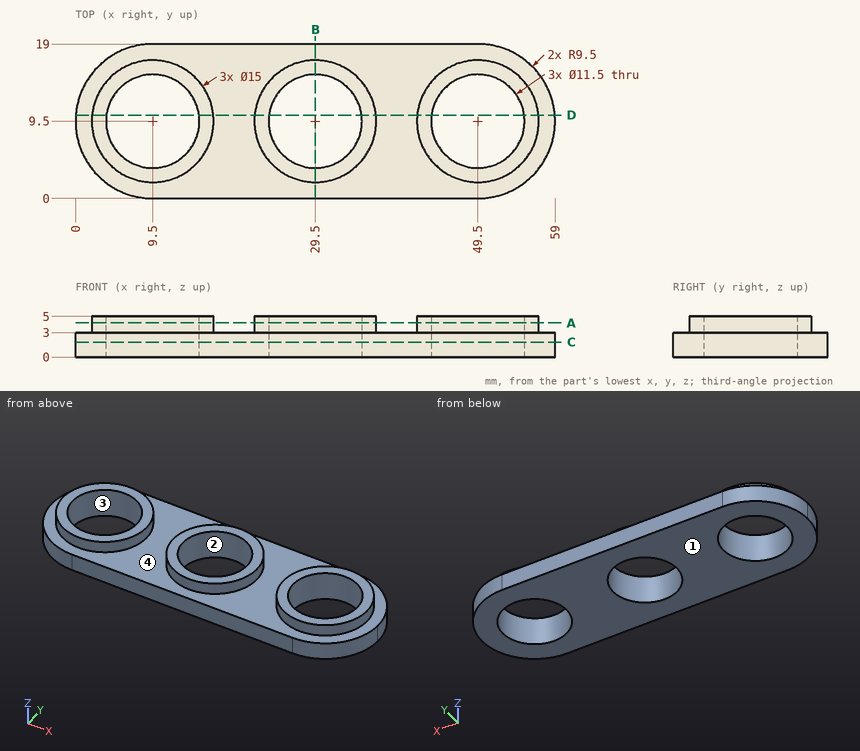
Verification items for this drawing (mm, ordinates from the low corner). A direction names the side the tool comes from. Coordinates: 2 decimals unless noted, no trailing zeros. Write each loop counter-clockwise with the first axis right and the second up, starting at its lowest first coordinate (ties: lowest second). Pieces come first, ordered by that corner, then holes. Notation, with made-up numbers: M -33.75,68.25 L 14.25,68.25 A18 ccw 14.25,78.25 Z; hole C -1,55 d11. An arc over 180 degrees is marked long. One line per item, written item: value. Start each with the question number.
(1) Depth check by flat-ended pin: pin 1 (2 mm diameter, centred on y = 9, z = 4.5, fed in from +X); pin 2 (10.5 mm diameter, centred on x = 9.5, y = 9.5, fed in from -Z); pin 3 (2 mm diameter, centred on y = 15, z = 3, fed in from -X); pin 4 (2 mm diameter, centred on y = 3, z = 3.5, fed in from +X). Enter the tip coordinate at first touch or a pass-through.
(2) Scan lines: line 1 along Y through (x, z) = (9.5, 1.6); line 2 along Y through (x, z) = (9.5, 3.3); line 3 along X through (y, z) = (8.25, 1.75). Record each from-to range of solid material in increasing order. Write a range as [from, to].
(3) Sectioned sample at B-B, the plane x = 29.5. Enter the section's corners in (y, z), and give its area (3 significant figures).
(4) Sectioned sample at A-A, the plane z = 4.2. Enter the section's corners in (x, y).
(5) Sectioned sample at D-D, the plane y = 10.25. Enter the section's corners in (x, z), and give its area (3 significant figures).
(6) Release check for a two-part mould opening along X. For the marked faces 1 and 2 record: released by +X, released by -X, zero draft, split by the parting line, or undercut.
(7) Sectioned sample at C-C, the plane z = 1.85. Enter the section's corners in (x, y), and give its area (3 significant figures).
(8) Tool access check on the marked faces 3 and 4. Record the directions out of +Z, -Z, +X, -X, +Y, -Y that give a thin tool (end or side, any length) a straight path to the whole face; none if there is none.
Filled sheet:
1. pin 1: x = 57
1. pin 2: through
1. pin 3: x = 1.13
1. pin 4: x = 57.15
2. line 1: [0, 3.75], [15.25, 19]
2. line 2: [2, 3.75], [15.25, 17]
2. line 3: [0.08, 3.89], [15.11, 23.89], [35.11, 43.89], [55.11, 58.92]
3. outline: M 0,0 L 3.75,0 L 3.75,5 L 2,5 L 2,3 L 0,3 Z; M 15.25,0 L 19,0 L 19,3 L 17,3 L 17,5 L 15.25,5 Z
3. area: 29.5 mm²
4. outline: C 9.5,9.5 d15; C 29.5,9.5 d15; C 49.5,9.5 d15; hole C 9.5,9.5 d11.5; hole C 29.5,9.5 d11.5; hole C 49.5,9.5 d11.5
5. outline: M 0.03,0 L 3.8,0 L 3.8,5 L 2.04,5 L 2.04,3 L 0.03,3 Z; M 15.2,0 L 23.8,0 L 23.8,5 L 22.04,5 L 22.04,3 L 16.96,3 L 16.96,5 L 15.2,5 Z; M 35.2,0 L 43.8,0 L 43.8,5 L 42.04,5 L 42.04,3 L 36.96,3 L 36.96,5 L 35.2,5 Z; M 55.2,0 L 58.97,0 L 58.97,3 L 56.96,3 L 56.96,5 L 55.2,5 Z
5. area: 95.3 mm²
6. face 1: zero draft
6. face 2: undercut
7. outline: M 9.5,0 L 49.5,0 A9.5 ccw 49.5,19 L 9.5,19 A9.5 ccw Z; hole C 9.5,9.5 d11.5; hole C 29.5,9.5 d11.5; hole C 49.5,9.5 d11.5
7. area: 732 mm²
8. face 3: +Z, -Z
8. face 4: +Z
